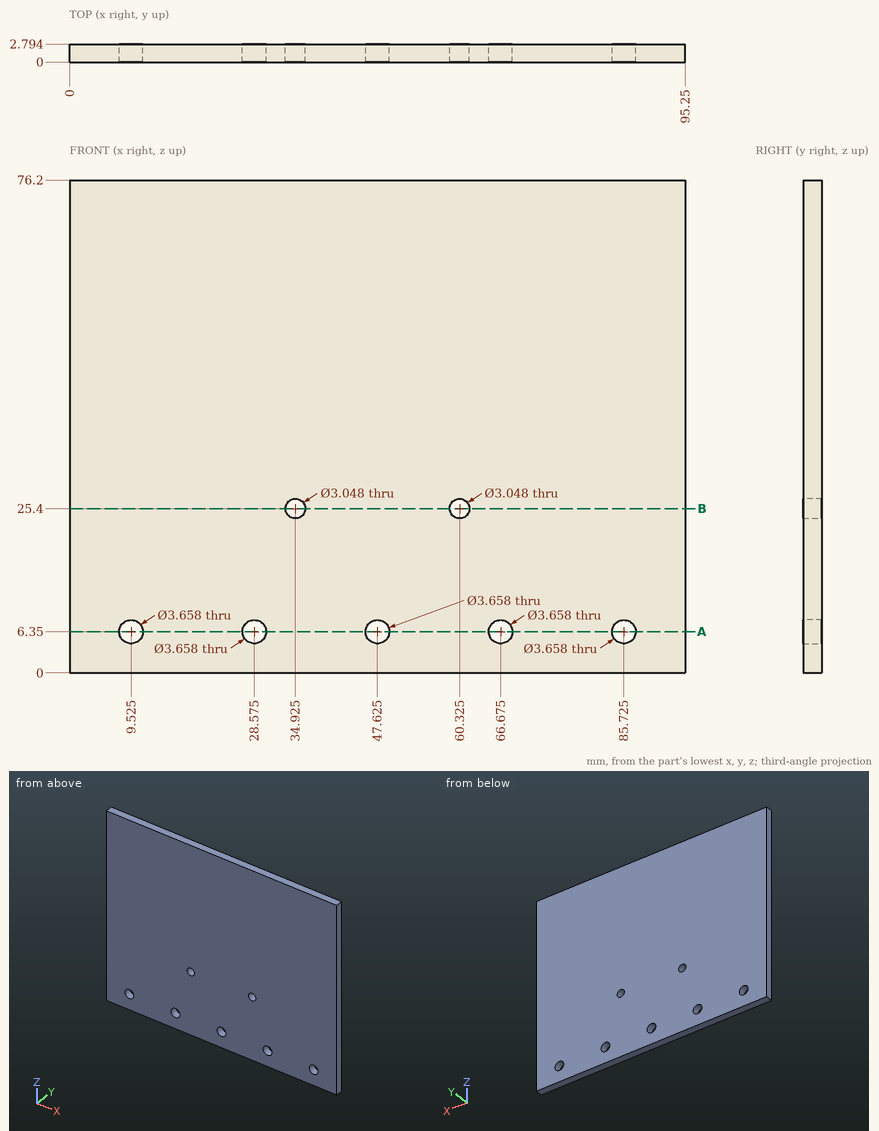
Can you work these out from the drawing? Everything is in mm from the part's minimum corner. Give positions to 0.01 mm unless a question says otherwise; leave off trailing zeros. Loops run counter-clockwise (first coordinate to the right, second up) from the corner with the lowest first, then second, coordinate; pieces in that order, holes last. Notation, with made-up numbers: (16, 49.5) -> (62, 49.5) arc R35 ccw to (62, 83.5) -> close; hole circle Ø6 at (-31.5, -35.75). An arc over 180 degrees is marked (long way). Return JSON: item names as keys, results as strings.
Item 1: I need wall thicknesses on L1, parallel to X at y = 1.9, z = 6.35; L2, parallel to Z at x = 86, y = 0.25; L3, parallel to Z at x = 65.5, y = 1.05. Which ranges of each line are inside material? Lowest first, please. Write a range as from..to.
Geometry results:
{"L1": "x = 0..7.7, 11.35..26.75, 30.4..45.8, 49.45..64.85, 68.5..83.9, 87.55..95.25", "L2": "z = 0..4.54, 8.16..76.2", "L3": "z = 0..4.95, 7.75..76.2"}
Item 2: If we section it at B-B on z = 25.4: List the corners of the cut face in (x, y) for me.
Geometry results:
{"outline": "(0, 0) -> (33.4, 0) -> (33.4, 2.79) -> (0, 2.79) -> close; (36.45, 0) -> (58.8, 0) -> (58.8, 2.79) -> (36.45, 2.79) -> close; (61.85, 0) -> (95.25, 0) -> (95.25, 2.79) -> (61.85, 2.79) -> close"}
Item 3: If we section it at A-A on z = 6.35: List the corners of the cut face in (x, y) for me.
Geometry results:
{"outline": "(0, 0) -> (7.7, 0) -> (7.7, 2.79) -> (0, 2.79) -> close; (11.35, 0) -> (26.75, 0) -> (26.75, 2.79) -> (11.35, 2.79) -> close; (30.4, 0) -> (45.8, 0) -> (45.8, 2.79) -> (30.4, 2.79) -> close; (49.45, 0) -> (64.85, 0) -> (64.85, 2.79) -> (49.45, 2.79) -> close; (68.5, 0) -> (83.9, 0) -> (83.9, 2.79) -> (68.5, 2.79) -> close; (87.55, 0) -> (95.25, 0) -> (95.25, 2.79) -> (87.55, 2.79) -> close"}
